Could you check a few things on this model? Use its own coordinates, in mm. Face numbers are marked on the shaded views. A direction names the side the tool comes from. Give positions to 0.01 mm unless a question says otherwise; leave off trailing zeros. Loops run counter-clockwise (first coordinate to the right, second up) from the corner with the lowest first, then second, coordinate; pieces in that order, holes last. Notation, with made-up numbers: M 60,39.25 L 96,39.25 A37 cw 96,77.25 Z; hole C 82,48 d5. An arc over 180 degrees is marked long. Use a Markdown table: item, result. Add a question column.
1) Suppose I cut it at D-D on y = -33. List the corners of the cut face in (x, z) for me, and give its area (3 significant figures).
2) We'd pull the mould along X, two halves only. Please class the marked faces 4, 5, 6 and 7: +X half, -X half, draft (parallel to the pull), parting line (faces both ways), or undercut.
3) If I drill on line 1 along Y through (x, z) = (55, 16.75); line 2 along X through (y, z) = (-36.5, 8.75); line 3 along Y through (x, z) = (20.5, 9.5), over which ranges is the centre line in solid material (lowest first)? Write a range as [from, to].
4) Will these pins go through, and if not, where does the flat tip stop? pin 1 Ø12 at (y, z) = (-103, 20) entering from +X; pin 2 Ø1.5 at (y, z) = (-38, 9) entering from +X; pin 3 Ø6.5 at (y, z) = (-110, 8.5) entering from +X; pin 4 Ø4.5 at (y, z) = (-112.5, 12.5) entering from +X.
5) Suppose I cut it at B-B on y = -112.5. List the corners of the cut face in (x, z) for me.
6) Which directions (+Z, -Z, +X, -X, +Y, -Y) give clear straight access to the entire face, cutting with the end or side of a thin tool? Please do the marked faces 1, 2 and 3.
7) Suppose I cut it at A-A on z = 12.5. List the corners of the cut face in (x, y) for me, and give its area (3 significant figures).
8) Suppose I cut it at C-C on x = 87. List the corners of the cut face in (y, z) for me, and give its area (3 significant figures).
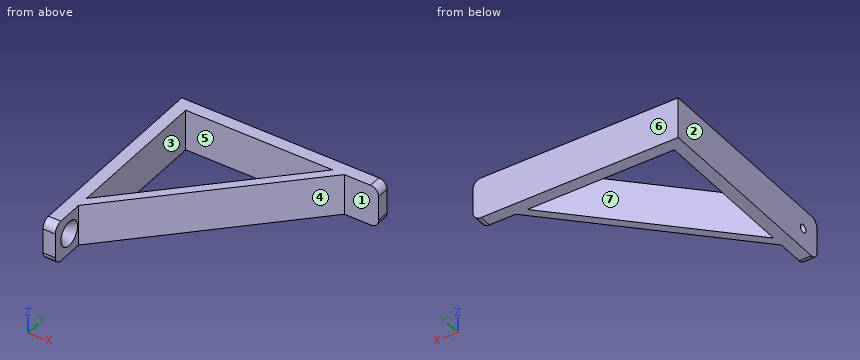
```python
from build123d import *

# Parameters (mm, degrees)
F0_W     = 117.5
F0_H     = 7.5
F0_W_2   = 7.5
F0_H_2   = 117.5
F1_DEPTH = 25
F3_DEPTH = 25
F4_R     = 2.5
F5_DEPTH = 25
F6_SIZE  = 5
F7_R     = 5


with BuildPart() as f1:
    # F0 (on Top) → F1 (new body)
    with BuildSketch(Plane.XY):
        with Locations((66.25, -3.75)):
            Rectangle(F0_W, F0_H)
        with Locations((3.75, -3.75)):
            Rectangle(F0_W_2, F0_H)
        with Locations((3.75, -66.25)):
            Rectangle(F0_W_2, F0_H_2)
    extrude(amount=F1_DEPTH)

    # F2 (on face) → F3 (join)
    with BuildSketch(Plane.XY.offset(25)):
        Polygon((96.9734936953, -7.5), (7.5, -96.9734936953), (7.5, -104.0445615071), (11.0355339059, -100.5090276012), (100.5090276012, -11.0355339059), (104.0445615071, -7.5), align=None)
    extrude(amount=-F3_DEPTH)

    # F4 (on face) → F5 (cut)
    with BuildSketch(Plane(origin=(0, 0, 0), x_dir=(0, -1, 0), z_dir=(-1, 0, 0))):
        with Locations((112.5, 12.5)):
            Circle(F4_R)
    extrude(amount=-F5_DEPTH, mode=Mode.SUBTRACT)

    # F6
    f6_edges = [f1.edges().sort_by_distance(p)[0] for p in [
        (7.5, -110, 12.5),
    ]]
    chamfer(f6_edges, length=F6_SIZE)

    # F7
    f7_edges = [f1.edges().sort_by_distance(p)[0] for p in [
        (3.75, -125, 25),
        (3.75, -125, 0),
        (125, -3.75, 25),
        (125, -3.75, 0),
    ]]
    fillet(f7_edges, radius=F7_R)


solid = f1.part
```
Answer block:
| question | item | result |
|---|---|---|
| 1 | outline | M 0,0 L 7.5,0 L 7.5,25 L 0,25 Z; M 71.47,0 L 78.54,0 L 78.54,25 L 71.47,25 Z |
| 1 | area | 364 mm^2 |
| 2 | face 4 | +X half |
| 2 | face 5 | undercut |
| 2 | face 6 | draft |
| 2 | face 7 | undercut |
| 3 | line 1 | y = [-56.54, -49.47], [-7.5, 0] |
| 3 | line 2 | x = [0, 7.5], [67.97, 75.04] |
| 3 | line 3 | y = [-91.04, -83.97], [-7.5, 0] |
| 4 | pin 1 | stops at x = 14.54 |
| 4 | pin 2 | stops at x = 74.29 |
| 4 | pin 3 | stops at x = 7.5 |
| 4 | pin 4 | passes through |
| 5 | outline | M 0,0 L 7.5,0 L 7.5,5 L 2.5,10 L 0,10 Z; M 0,15 L 2.5,15 L 7.5,20 L 7.5,25 L 0,25 Z |
| 6 | face 1 | +Z, -Z, +X, -Y |
| 6 | face 2 | +Z, -Z, -X, +Y, -Y |
| 6 | face 3 | +Z, -Z |
| 7 | outline | M 0,-125 L 7.5,-125 L 7.5,-120 L 2.5,-115 L 0,-115 Z; M 0,-110 L 2.5,-110 L 7.5,-105 L 7.5,-104.04 L 104.04,-7.5 L 125,-7.5 L 125,0 L 0,0 Z; hole M 7.5,-96.97 L 96.97,-7.5 L 7.5,-7.5 Z |
| 7 | area | 2,410 mm^2 |
| 8 | outline | M -24.54,0 L -17.47,0 L -17.47,25 L -24.54,25 Z; M -7.5,0 L 0,0 L 0,25 L -7.5,25 Z |
| 8 | area | 364 mm^2 |
